Read the model definition and answer for the solid it produces. Units are mm, in the model's axes. Round coordinates to 2 decimals unless told otherwise and drop trailing zeros.
from build123d import *

# Parameters (mm, degrees)
BOSS_EXTRUDE1_DEPTH = 350
CIRPATTERN1_COUNT   = 4


with BuildPart() as part:
    # Sketch1 → Boss-Extrude1 (new, symmetric)
    with BuildSketch(Plane(origin=(0, 0, 0), x_dir=(0, -1, 0), z_dir=(0, 0, 1))):
        with BuildLine():
            Line((0, 5.3), (0, 3.65))
            ThreePointArc((0, 3.65), (-2.580939751, 2.580939751), (-3.65, 0))
            Line((-3.65, 0), (-5.3, 0))
            Line((-5.3, 0), (-6, 1.25))
            Line((-6, 1.25), (-6, 4.232224593))
            Line((-6, 4.232224593), (-10.01775891, 8.249983504))
            Line((-10.01775891, 8.249983504), (-12.68, 8.249983504))
            Line((-12.68, 8.249983504), (-12.68, 4.549990808))
            ThreePointArc((-12.68, 4.549990808), (-12.826446609, 4.196437418), (-13.18, 4.049990808))
            Line((-13.18, 4.049990808), (-14.5, 4.049990808))
            ThreePointArc((-14.5, 4.049990808), (-14.853553391, 4.196437418), (-15, 4.549990808))
            Line((-15, 4.549990808), (-15, 13))
            Line((-15, 13), (-13, 15))
            Line((-13, 15), (-4.549990808, 15))
            ThreePointArc((-4.549990808, 15), (-4.196437418, 14.853553391), (-4.049990808, 14.5))
            Line((-4.049990808, 14.5), (-4.049990808, 13.18))
            ThreePointArc((-4.049990808, 13.18), (-4.196437418, 12.826446609), (-4.549990808, 12.68))
            Line((-4.549990808, 12.68), (-8.249983504, 12.68))
            Line((-8.249983504, 12.68), (-8.249983504, 10.01775891))
            Line((-8.249983504, 10.01775891), (-4.232224593, 6))
            Line((-4.232224593, 6), (-1.25, 6))
            Line((-1.25, 6), (0, 5.3))
        make_face()
        with BuildLine():
            Line((-10.5, 9.5), (-12.7, 9.5))
            ThreePointArc((-12.7, 9.5), (-13.407106781, 9.792893219), (-13.7, 10.5))
            Line((-13.7, 10.5), (-13.7, 12.461522369))
            Line((-13.7, 12.461522369), (-12.461522369, 13.7))
            Line((-12.461522369, 13.7), (-10.5, 13.7))
            ThreePointArc((-10.5, 13.7), (-9.792893219, 13.407106781), (-9.5, 12.7))
            Line((-9.5, 12.7), (-9.5, 10.5))
            ThreePointArc((-9.5, 10.5), (-9.792893219, 9.792893219), (-10.5, 9.5))
        make_face(mode=Mode.SUBTRACT)
    boss_extrude1 = extrude(amount=BOSS_EXTRUDE1_DEPTH, both=True)

    # CirPattern1: Boss-Extrude1 ×4 about axis
    cirpattern1_axis = Axis((0, 0, 0), (0, 0, 1))
    for i in range(1, CIRPATTERN1_COUNT):
        add(boss_extrude1.rotate(cirpattern1_axis, i * 360 / CIRPATTERN1_COUNT))


solid = part.part
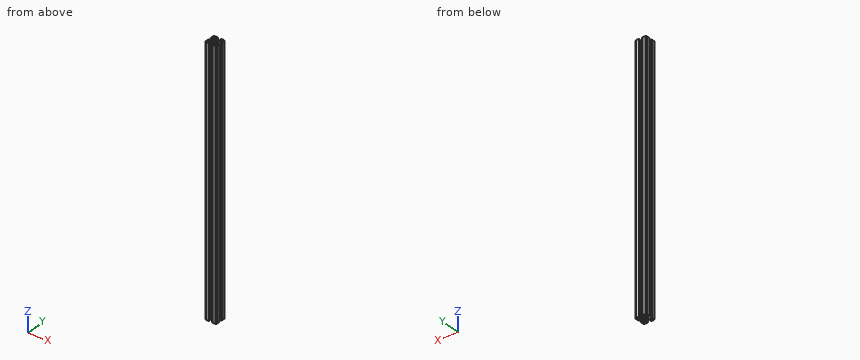
Q1. Section A-A (z = 69.5) is taken. State how many separate pieces and enclosed holes the cut face has, then the cut area to 3 significant figures.
Verdict:
separate pieces: 1
enclosed holes: 5
area: 329 mm2
Q2. Straight lines are drawn through the part: probe 1 along Y at (x, z) = (-11.75, 303); probe 2 along Y at (x, z) = (-13.5, -117). For each, find the intervals that lie inside material, in ascending order.
Verdict:
probe 1: y = -15 to -13.7, -9.5 to -8.25, 8.25 to 9.5, 13.7 to 15
probe 2: y = -14.5 to -12.66, -9.9 to -4.05, 4.05 to 9.9, 12.66 to 14.5
Q3. Flat-ended cylindrical pins translate along their axes: pin 1 Ø1.5 at (x, z) = (1.5, -59) entering from -Y; pin 2 Ø8 at (x, z) = (-0.5, 192.5) entering from -Y; pin 3 Ø0.9 at (y, z) = (-2.5, -8.5) entering from +X. Find the tip coordinate at first contact, or state that the pin passes through.
Verdict:
pin 1: stops at y = -6
pin 2: stops at y = -15
pin 3: stops at x = 6
